```python
from build123d import *

# Parameters (mm, degrees)
F0_R     = 11.2
F1_DEPTH = 0.25


with BuildPart() as f1:
    # F0 (on Top) → F1 (new body)
    with BuildSketch(Plane.XY):
        with BuildLine():
            ThreePointArc((11.243032, 24.633988), (12.553076, 27.781021), (13, 31.160414))
            ThreePointArc((13, 31.160414), (11.172924, 37.806147), (6.205266, 42.58384))
            ThreePointArc((6.205266, 42.58384), (-11.321974, 37.548911), (-6.570071, 19.942831))
            ThreePointArc((-6.570071, 19.942831), (3.310722, 18.589053), (11.243032, 24.633988))
        make_face()
        with Locations((0, 31.160414)):
            Circle(F0_R, mode=Mode.SUBTRACT)
        with BuildLine():
            ThreePointArc((6.205266, 42.58384), (11.172924, 37.806147), (13, 31.160414))
            ThreePointArc((13, 31.160414), (12.553076, 27.781021), (11.243032, 24.633988))
            ThreePointArc((11.243032, 24.633988), (20.16491, 22.206844), (25.685808, 14.789929))
            ThreePointArc((25.685808, 14.789929), (21.662594, 32.693926), (6.205266, 42.58384))
        make_face()
        with BuildLine():
            ThreePointArc((20.433129, -4.352398), (12.296612, 9.017977), (11.243032, 24.633988))
            ThreePointArc((11.243032, 24.633988), (3.310722, 18.589053), (-6.570071, 19.942831))
            ThreePointArc((-6.570071, 19.942831), (-14.190564, 6.359224), (-26.944847, -2.580271))
            ThreePointArc((-26.944847, -2.580271), (-17.778886, -6.402277), (-13.98571, -15.580207))
            ThreePointArc((-13.98571, -15.580207), (-13.985915, -15.653237), (-13.98653, -15.726265))
            ThreePointArc((-13.98653, -15.726265), (1.62392, -15.259159), (15.697868, -22.028821))
            ThreePointArc((15.697868, -22.028821), (14.428475, -12.216303), (20.433129, -4.352398))
        make_face()
        Circle(F0_R, mode=Mode.SUBTRACT)
        with BuildLine():
            ThreePointArc((39.98571, -15.580207), (33.459366, -4.306708), (20.433129, -4.352398))
            ThreePointArc((20.433129, -4.352398), (14.428475, -12.216303), (15.697868, -22.028821))
            ThreePointArc((15.697868, -22.028821), (15.707601, -22.036816), (15.717332, -22.044815))
            ThreePointArc((15.717332, -22.044815), (15.714954, -22.049655), (15.712573, -22.054494))
            ThreePointArc((15.712573, -22.054494), (23.767322, -28.175523), (33.771118, -26.668861))
            ThreePointArc((33.771118, -26.668861), (38.326131, -21.935901), (39.98571, -15.580207))
        make_face()
        with Locations((26.98571, -15.580207)):
            Circle(F0_R, mode=Mode.SUBTRACT)
        with BuildLine():
            ThreePointArc((-13.98571, -15.580207), (-17.778886, -6.402277), (-26.944847, -2.580271))
            ThreePointArc((-26.944847, -2.580271), (-36.271667, -6.48235), (-39.982088, -15.88706))
            ThreePointArc((-39.982088, -15.88706), (-26.9053, -28.579958), (-13.98653, -15.726265))
            ThreePointArc((-13.98653, -15.726265), (-13.985915, -15.653237), (-13.98571, -15.580207))
        make_face()
        with Locations((-26.98571, -15.580207)):
            Circle(F0_R, mode=Mode.SUBTRACT)
        with BuildLine():
            ThreePointArc((-39.982088, -15.88706), (-36.271667, -6.48235), (-26.944847, -2.580271))
            ThreePointArc((-26.944847, -2.580271), (-29.303818, 6.359874), (-25.641029, 14.849569))
            ThreePointArc((-25.641029, 14.849569), (-39.12779, 2.428274), (-39.982088, -15.88706))
        make_face()
        with BuildLine():
            ThreePointArc((15.717332, -22.044815), (15.707601, -22.036816), (15.697868, -22.028821))
            ThreePointArc((15.697868, -22.028821), (15.705213, -22.041661), (15.712573, -22.054494))
            ThreePointArc((15.712573, -22.054494), (15.714954, -22.049655), (15.717332, -22.044815))
        make_face()
        with BuildLine():
            ThreePointArc((-0.029261, -29.630596), (17.47986, -35.099075), (33.771118, -26.668861))
            ThreePointArc((33.771118, -26.668861), (23.767322, -28.175523), (15.712573, -22.054494))
            ThreePointArc((15.712573, -22.054494), (9.149566, -28.560156), (-0.029261, -29.630596))
        make_face()
    extrude(amount=F1_DEPTH)


solid = f1.part
```
Geometry: final body of the model. Coordinates: model frame, mm. Coordinates: 2 decimals unless noted, no trailing zeros. Order: outer loops, then holes, each group sorted by start corner. A loop starts at its lowest first (then second) coordinate and runs counter-clockwise, first axis right, second up.
Item 1: Material intervals for line 1 along X through (y, z) = (4.5, 0.15); line 2 along X through (y, z) = (22, 0.1); line 3 along Y through (x, z) = (2, 0.15), sorted ascending.
Answer:
line 1: x = -38.04 to -29.32, -16 to -10.26, 10.26 to 14.11
line 2: x = -9.22 to -6.44, 6.44 to 10.89, 20.46 to 25.82
line 3: y = -31.14 to -29.92, -15.34 to -11.02, 11.02 to 20.14, 42.18 to 44.01
Item 2: Section query D-D (y = 23). Output: boundary loops of the cut face in (x, z).
Answer:
outline: (-10.12, 0) - (-7.67, 0) - (-7.67, 0.25) - (-10.12, 0.25) - close; (7.67, 0) - (11, 0) - (11, 0.25) - (7.67, 0.25) - close; (18.85, 0) - (25.67, 0) - (25.67, 0.25) - (18.85, 0.25) - close
Item 3: Section query B-B (x = 14). Output: boundary loops of the cut face in (y, z), then the cut area to 3 significant figures.
Answer:
outline: (-35.15, 0) - (-24.73, 0) - (-24.73, 0.25) - (-35.15, 0.25) - close; (-20.72, 0) - (4.72, 0) - (4.72, 0.25) - (-20.72, 0.25) - close; (24.55, 0) - (39.72, 0) - (39.72, 0.25) - (24.55, 0.25) - close
area: 12.8 mm2
Item 4: Section query A-A (y = -19). Output: boundary loops of the cut face in (x, z).
Answer:
outline: (-39.53, 0) - (-37.65, 0) - (-37.65, 0.25) - (-39.53, 0.25) - close; (-16.32, 0) - (-14.44, 0) - (-14.44, 0.25) - (-16.32, 0.25) - close; (11.33, 0) - (16.32, 0) - (16.32, 0.25) - (11.33, 0.25) - close; (37.65, 0) - (39.53, 0) - (39.53, 0.25) - (37.65, 0.25) - close
Item 5: Section query C-C (x = 2). Output: boundary loops of the cut face in (y, z).
Answer:
outline: (-31.14, 0) - (-29.92, 0) - (-29.92, 0.25) - (-31.14, 0.25) - close; (-15.34, 0) - (-11.02, 0) - (-11.02, 0.25) - (-15.34, 0.25) - close; (11.02, 0) - (20.14, 0) - (20.14, 0.25) - (11.02, 0.25) - close; (42.18, 0) - (44.01, 0) - (44.01, 0.25) - (42.18, 0.25) - close
